Build history of the part. All positions in model axes, mm. A direction names the side the tool comes from. Coordinates: 2 decimals unless noted, no trailing zeros. Loops run counter-clockwise (first coordinate to the right, second up) from the corner with the lowest first, then second, coordinate; pieces in that order, holes last. Notation, with made-up numbers: (19.5, 54.5) - (29.5, 54.5) arc R8 ccw to (29.5, 65.5) - close; hole circle Ø9 at (53.25, -2). An arc over 180 degrees is marked (long way). One line per item, written item: value.
```python
from build123d import *

# Parameters (mm, degrees)
SKETCH_1_W          = 8
SKETCH_1_H          = 8
EXTRUDE_1_DEPTH     = 20
SKETCH_2_R          = 1.6
CUT_EXTRUDE_1_DEPTH = 23.978250586
SKETCH_4_W          = 2
SKETCH_4_H          = 8
EXTRUDE_3_DEPTH     = 10
SKETCH_5_W          = 5.2
SKETCH_5_H          = 8.5
CUT_EXTRUDE_2_DEPTH = 24.748684174
FILLET_1_R          = 3
SKETCH_6_R          = 1.45
CUT_EXTRUDE_3_DEPTH = 25.657656012
FILLET_2_R          = 3


with BuildPart() as part:
    # 草图1 → 凸台-拉伸1 (new body)
    with BuildSketch(Plane(origin=(0, 0, 0), x_dir=(1, 0, 0), z_dir=(0, 1, 0))):
        with Locations((4, -4)):
            Rectangle(SKETCH_1_W, SKETCH_1_H)
    extrude(amount=EXTRUDE_1_DEPTH)

    # 草图2 → 切除-拉伸1 (cut, through all)
    with BuildSketch(Plane.XY.offset(8)):
        with Locations((4, 4)):
            Circle(SKETCH_2_R)
    extrude(amount=-CUT_EXTRUDE_1_DEPTH, mode=Mode.SUBTRACT)

    # 草图4 → 凸台-拉伸3 (add)
    with BuildSketch(Plane(origin=(0, 20, 0), x_dir=(1, 0, 0), z_dir=(0, 1, 0))):
        with Locations((-1, -4)):
            Rectangle(SKETCH_4_W, SKETCH_4_H)
        with Locations((9, -4)):
            Rectangle(SKETCH_4_W, SKETCH_4_H)
    extrude(amount=-EXTRUDE_3_DEPTH)

    # 草图5 → 切除-拉伸2 (cut, through all)
    with BuildSketch(Plane.XY.offset(8)):
        with Locations((4, 15.75)):
            Rectangle(SKETCH_5_W, SKETCH_5_H)
    extrude(amount=-CUT_EXTRUDE_2_DEPTH, mode=Mode.SUBTRACT)

    # 圆角1
    # the kernel refuses this fillet: 3 mm, written as the material it adds along each edge
    with BuildSketch(Plane(origin=(8, 10, 8), x_dir=(0, -1, 0), z_dir=(0, 0, -1))) as fillet_1_piece_1:
        with BuildLine():
            CenterArc((2.828427125, -3), FILLET_1_R, 90, 70.528779366)
            Line((0, -2), (-0.056568542, -1.98))
            ThreePointArc((-0.056568542, -1.98), (-0.06, -1), (-0.06, 0))
            Line((-0.06, 0), (0, 0.06))
            Line((0, 0.06), (2.828427125, 0.06))
            Line((2.828427125, 0.06), (2.828427125, 0))
        make_face()
    extrude(amount=8)
    with BuildSketch(Plane(origin=(0, 10, 8), x_dir=(-1, 0, 0), z_dir=(0, 0, -1))) as fillet_1_piece_2:
        with BuildLine():
            CenterArc((3, -2.828427125), FILLET_1_R, 109.471220634, 70.528779366)
            Line((0, -2.828427125), (-0.06, -2.828427125))
            Line((-0.06, -2.828427125), (-0.06, 0))
            Line((-0.06, 0), (0, 0.06))
            ThreePointArc((0, 0.06), (1, 0.06), (1.98, 0.056568542))
            Line((1.98, 0.056568542), (2, 0))
        make_face()
    extrude(amount=8)

    # 草图6 → 切除-拉伸3 (cut, through all)
    with BuildSketch(Plane(origin=(10, 0, 0), x_dir=(0, 0, -1), z_dir=(1, 0, 0))):
        with Locations((-4, 16)):
            Circle(SKETCH_6_R)
    extrude(amount=-CUT_EXTRUDE_3_DEPTH, mode=Mode.SUBTRACT)

    # 圆角2
    fillet_2_edges = [part.edges().sort_by_distance(p)[0] for p in [
        (8.3, 20, 0),
        (-2, 10, 4),
        (10, 10, 4),
        (-0.3, 20, 0),
        (8.3, 20, 8),
        (8, 0, 4),
        (0, 0, 4),
        (-0.3, 20, 8),
    ]]
    fillet(fillet_2_edges, radius=FILLET_2_R)


solid = part.part
```
Item 1: Pull direction Z, two halves, no side cores. Call faces 6 (the face through (-0.28, 16.98, 5.07)), 7 (the face through (4, 9, 8)), 8 (the face through (-2, 14, 4)): released by +Z, released by -Z, zero draft, split by the parting line, or undercut.
Check result:
face 6: undercut
face 7: released by +Z
face 8: zero draft
Item 2: Tool access for faces 1 (the face through (0, 20, 4)), 2 (the face through (8.32, 19.1, 0.86)), 3 (the face through (8, 5, 4)), 4 (the face through (4, 11.5, 4)), 5 (the face through (0, 5, 4)): list every direction of +Z, -Z, +X, -X, +Y, -Y with a clear straight run to the whole face (end or side of a thin tool).
Check result:
face 1: +Z, -Z, +X, -X, +Y
face 2: -Z, +X, -X, +Y
face 3: +Z, -Z, +X, -Y
face 4: +Z, -Z, +Y
face 5: +Z, -Z, -X, -Y
Item 3: Probe probe 1 along X at (y, z) = (18.5, 1); probe 2 along Y at (x, z) = (4, 2.5); probe 3 along Z at (x, y) = (9.75, 15.25). List the from-to ranges inside material, lowest first. Write a range as from..to.
Check result:
probe 1: x = -2..1.4, 6.6..10
probe 2: y = 0..2.4, 5.6..11.5
probe 3: z = 0..2.76, 5.24..8
Item 4: Cut at B-B, the plane y = 16. Write the cut outline in (x, z), then the cut area to 3 significant figures.
Check result:
outline: (-2, 0) - (1.4, 0) - (1.4, 2.55) - (-2, 2.55) - close; (-2, 5.45) - (1.4, 5.45) - (1.4, 8) - (-2, 8) - close; (6.6, 0) - (10, 0) - (10, 2.55) - (6.6, 2.55) - close; (6.6, 5.45) - (10, 5.45) - (10, 8) - (6.6, 8) - close
area: 34.7 mm^2
Item 5: Cut at A-A, the plane z = 4. Write the cut outline in (x, y).
Check result:
outline: (-2, 11.64) arc R3 ccw to (-1, 9.41) arc R3 cw to (0, 7.17) - (0, 3) arc R3 ccw to (3, 0) - (5, 0) arc R3 ccw to (8, 3) - (8, 7.17) arc R3 cw to (9, 9.41) arc R3 ccw to (10, 11.64) - (10, 14.55) - (6.6, 14.55) - (6.6, 11.5) - (1.4, 11.5) - (1.4, 14.55) - (-2, 14.55) - close; (-2, 17.45) - (1.4, 17.45) - (1.4, 20) - (-2, 20) - close; (6.6, 17.45) - (10, 17.45) - (10, 20) - (6.6, 20) - close; hole circle Ø3.2 at (4, 4)
Item 6: Drop flat-ended pins along their axis: P1, Ø4, axis at x = 3.5, z = 4, coming from the +Y side; P2, Ø1.9, axis at x = 4, y = 4, coming from the -Z side; P3, Ø1, axis at y = 10.5, z = 7, coming from the -X side; P4, Ø3.5, axis at y = 5, z = 4.5, coming from the -X side. Give the stop position or say it passes through.
Check result:
P1: stops at y = 11.5
P2: passes through
P3: stops at x = -1.93
P4: stops at x = 0
Item 7: Cut at D-D, the plane y = 18. Write the cut outline in (x, z).
Check result:
outline: (-2, 0.17) - (1.4, 0.17) - (1.4, 7.83) - (-2, 7.83) - close; (6.6, 0.17) - (10, 0.17) - (10, 7.83) - (6.6, 7.83) - close
Item 8: Cut at C-C, the plane x = 4. Write the cut outline in (y, z), then the cut area to 3 significant figures.
Check result:
outline: (0, 0) - (2.4, 0) - (2.4, 8) - (0, 8) - close; (5.6, 0) - (11.5, 0) - (11.5, 8) - (5.6, 8) - close
area: 66.4 mm^2
